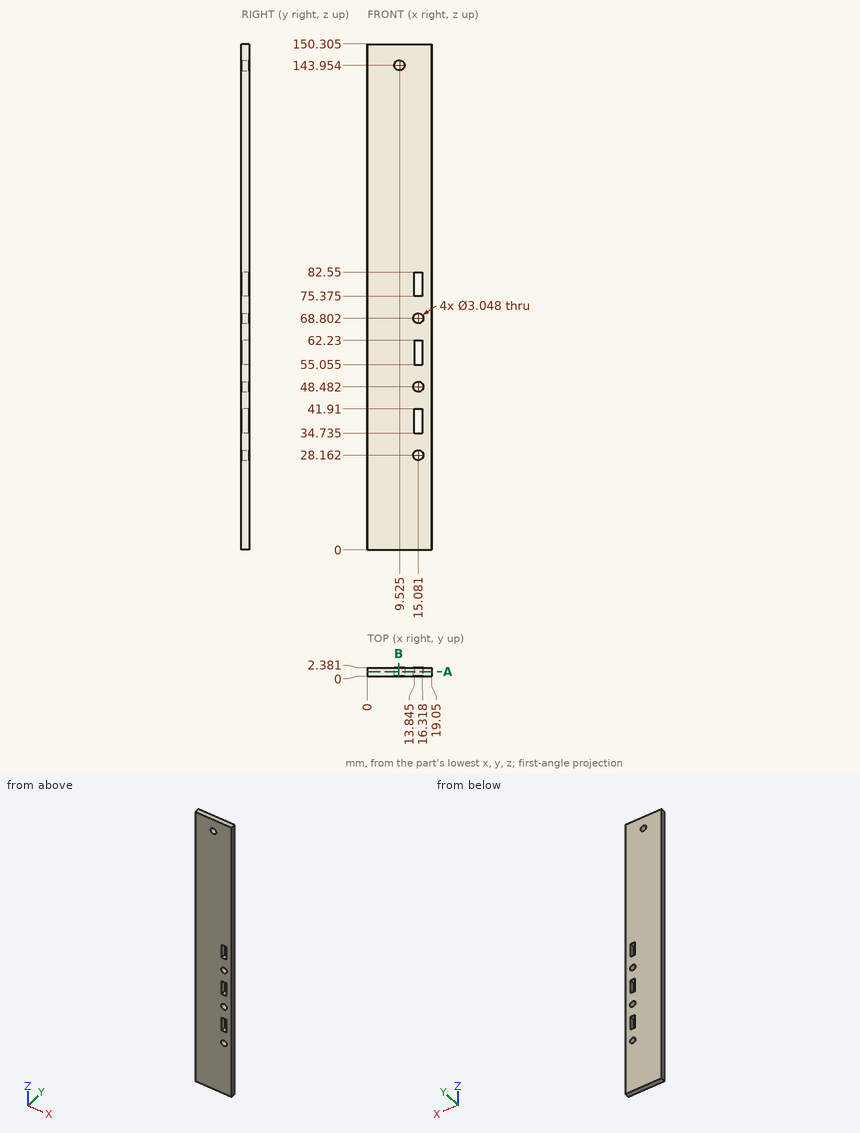
Can you work these out from the drawing? Everything is in mm from the part's minimum corner. Coordinates: 2 decimals unless noted, no trailing zeros. Loops run counter-clockwise (first coordinate to the right, second up) from the corner with the lowest first, then second, coordinate; pieces in that order, holes last. Notation, with made-up numbers: (-25, 80) - (18, 80) arc R31 ccw to (18, 117) - close; hole circle Ø6 at (52, 67.25). An arc over 180 degrees is marked (long way). Use a Markdown table: item, result.
Item 1: Will this pin go through, and if not, where does the flat tip stop? pin 1 (2.5 mm diameter, centred on x = 15.08, z = 68.8, fed in from +Y).
Numbers:
| item | result |
|---|---|
| pin 1 | passes through |
Item 2: I want a section at B-B on x = 9.25. Please give me the cut outline in (y, z) (1 decimal).
Numbers:
| item | result |
|---|---|
| outline | (0, 0) - (2.4, 0) - (2.4, 142.5) - (0, 142.5) - close; (0, 145.5) - (2.4, 145.5) - (2.4, 150.3) - (0, 150.3) - close |
Item 3: I want a section at A-A on y = 1.3. Give the number of separate pieces and of enclosed holes in the cut face, and give its area (3 significant figures).
Numbers:
| item | result |
|---|---|
| separate pieces | 1 |
| enclosed holes | 7 |
| area | 2,780 mm2 |
Item 4: If I drill on probe 1 along Z at (x, y) = (9.25, 0.5) (1 decimal); probe 2 along Z at (x, y) = (8.5, 1) (1 decimal), over which ranges is the centre line in solid material (lowest first)? Write a range as from..to.
Numbers:
| item | result |
|---|---|
| probe 1 | z = 0..142.5, 145.5..150.3 |
| probe 2 | z = 0..142.8, 145.1..150.3 |
